Could you check a few things on this model? Use its own coordinates, in mm. A direction names the side the tool comes from. Give positions to 0.01 mm unless a question says otherwise; leave off trailing zeros. Write each loop counter-clockwise with the first axis right and the second up, starting at its lowest first coordinate (ties: lowest second). Pieces come first, ordered by that corner, then holes. Notation, with made-up numbers: M 73.25,-38 L 107.25,-38 A28 cw 107.25,-4 Z; hole C -7,0 d7. An arc over 180 degrees is marked long. Answer as CSV lines item,"result". Start each with the question number.
from build123d import *

# Parameters (mm, degrees)
EXTRUDE_1_DEPTH     = 53
SKETCH_2_R          = 5
CUT_EXTRUDE_1_DEPTH = 75.01351228


with BuildPart() as part:
    # 草图1 → 凸台-拉伸1 (new, symmetric)
    with BuildSketch(Plane.XY):
        with BuildLine():
            Line((0, 1), (0, 37))
            ThreePointArc((0, 37), (0.292893219, 37.707106781), (1, 38))
            Line((1, 38), (2, 38))
            ThreePointArc((2, 38), (2.707106781, 37.707106781), (3, 37))
            Line((3, 37), (3, 8))
            ThreePointArc((3, 8), (4.464466094, 4.464466094), (8, 3))
            Line((8, 3), (37, 3))
            ThreePointArc((37, 3), (37.707106781, 2.707106781), (38, 2))
            Line((38, 2), (38, 1))
            ThreePointArc((38, 1), (37.707106781, 0.292893219), (37, 0))
            Line((37, 0), (1, 0))
            ThreePointArc((1, 0), (0.292893219, 0.292893219), (0, 1))
        make_face()
    extrude(amount=EXTRUDE_1_DEPTH, both=True)

    # 草图2 → 切除-拉伸1 (cut, through all)
    with BuildSketch(Plane(origin=(0, 3, 0), x_dir=(1, 0, 0), z_dir=(0, 1, 0))):
        with Locations(Location((21, 0, 0), (0, 0, 270))):
            Circle(SKETCH_2_R)
    extrude(amount=-CUT_EXTRUDE_1_DEPTH, mode=Mode.SUBTRACT)


solid = part.part
1. Imagine slicing it at A-A, the plane z = 0. Please give me the cut outline in (x, y), plus the area to 3 significant figures.
2. Imagine slicing it at C-C, the plane z = -42. Please give me the cut outline in (x, y).
3. Imagine slicing it at B-B, the plane x = 21. Please give me the cut outline in (y, z).
4. Thinking about a two-plate mould opening in X: for faces 3 (the flat face through (11, 2, -53)), 4 (the flat face through (3, 23, 1)), 5 (the cylindrical face through (16.12, 1.52, -1.08)), which applies, pulls with the +X half, pulls with the -X half, needs draft (parallel to the pull), parting line crosses it, or undercut?
5. Please list where these lines run through material, in increasing order: line 1 (X direction, y = 2.1, z = 0); line 2 (Y direction, x = 27, z = -47).
6. Will these pins go through, and if not, where does the flat tip stop? P1, Ø14.5, axis at y = 23.5, z = -22, coming from the +X side; P2, Ø8.5, axis at x = 29.5, z = -9.5, coming from the +Y side.
7. On a 3-axis mill with a long thin cutter (end or side, diameter ignored), from which of +Z, -Z, +X, -X, +Y, -Y can I reach the whole of each face in a straight line? I mean faces 1 (the flat face through (0, 19, 1)), 2 (the flat face through (29, 3, 1)). Say none if no direction works.
8. Imagine slicing it at D-D, the plane x = 14. Please give me the cut outline in (y, z), plus the area to 3 significant figures.
Solutions:
1,outline,"M 0,1 A1 ccw 1,0 L 16,0 L 16,3 L 8,3 A5 cw 3,8 L 3,37 A1 ccw 2,38 L 1,38 A1 ccw 0,37 Z; M 26,0 L 37,0 A1 ccw 38,1 L 38,2 A1 ccw 37,3 L 26,3 Z"
1,area,"193 mm²"
2,outline,"M 0,1 A1 ccw 1,0 L 37,0 A1 ccw 38,1 L 38,2 A1 ccw 37,3 L 8,3 A5 cw 3,8 L 3,37 A1 ccw 2,38 L 1,38 A1 ccw 0,37 Z"
3,outline,"M 0,-53 L 3,-53 L 3,-5 L 0,-5 Z; M 0,5 L 3,5 L 3,53 L 0,53 Z"
4,face 3,"needs draft"
4,face 4,"pulls with the +X half"
4,face 5,"undercut"
5,line 1,"0 to 16, 26 to 37.99"
5,line 2,"0 to 3"
6,P1,"x = 3"
6,P2,"y = 3"
7,face 1,"+Z, -Z, -X, +Y, -Y"
7,face 2,"+Z, -Z, +X, +Y"
8,outline,"M 0,-53 L 3,-53 L 3,53 L 0,53 Z"
8,area,"318 mm²"
